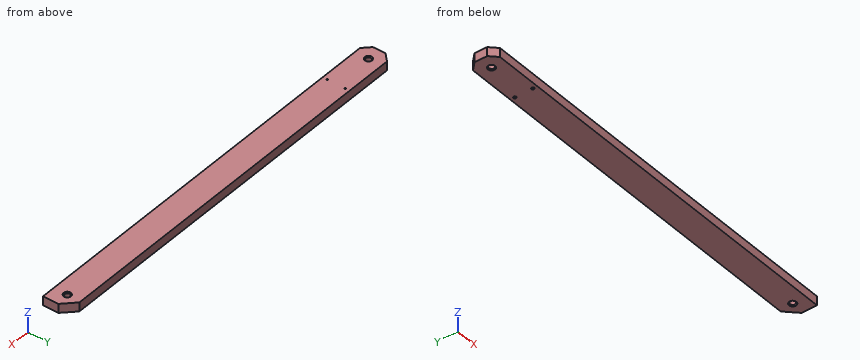
Autodesk Inventor part; units mm, degrees
ref_plane "YZ Plane" through (0, 0, 0) normal (1, 0, 0) x (0, 1, 0)
ref_plane "XZ Plane" through (0, 0, 0) normal (0, 1, 0) x (-1, 0, 0)
ref_plane "XY Plane" through (0, 0, 0) normal (0, 0, 1) x (1, 0, 0)
sketch "Sketch1" plane through (0, 0, 0) normal (0, 0, 1) x (1, 0, 0)
  line L0 (0, 0) -> (2250, 0)
  line L1 (2250, 0) -> (2250, 150)
  line L2 (2250, 150) -> (0, 150)
  line L3 (0, 150) -> (0, 0)
  dimension "d0" = 150
  dimension "d1" = 2250
extrude "Extrusion1" add sketch "Sketch1" along normal blind 50
sketch "Sketch2" plane through (0, 0, 50) normal (0, 0, 1) x (1, 0, 0)
  line L0 (0, 150) -> (0, 0)
  line L1 (2250, 0) -> (2250, 150)
  point P0 (75, 75)
  point P1 (2175, 75)
  point P2 (0, 75)
  dimension "d4" = 75
  dimension "d5" = 75
hole "Hole1" at (75, 75, 50) at (2175, 75, 50) direction (0, 0, -1) diameter 30 end through all
chamfer "Chamfer1" distance 5 angle 45 4 edges at (75, 90, 50) (2175, 90, 50) (75, 90, 0) (2175, 90, 0)
chamfer "Chamfer2" distance 65 angle 45 1 edges at (2250, 150, 25) measured on face at (2250, 50, 16.6667)
chamfer "Chamfer3" distance 40 angle 45 2 edges at (0, 150, 25) (0, 0, 25)
sketch "Sketch3" plane through (0, 0, 0) normal (0, 0, -1) x (-1, 0, 0)
  line L0 (-40, 0) -> (-2250, 0)
  line L1 (-2185, 150) -> (-40, 150)
  line L2 (0, 110) -> (0, 40)
  point P0 (0, 0)
  point P1 (-300, 25)
  point P2 (-300, 125)
  dimension "d22" = 25
  dimension "d23" = 25
  dimension "d24" = 300
hole "Hole2" at (300, 25, 0) at (300, 125, 0) direction (0, 0, 1) diameter 8.433 end through all countersink diameter 16.129 countersink angle 82
properties part number "Top_Rear Plank_LHS" material "Wood (Birch)"
The model under review builds one solid part; all positions refer to its coordinate system, in mm. Give positions to 0.01 mm unless a question says otherwise; leave off trailing zeros. Order: outer loops, then holes, each group sorted by start corner. A loop starts at its lowest first (then second) coordinate and runs counter-clockwise, first axis right, second up. Notation, with made-up numbers: M 29.5,48 L 46.5,48 A9 cw 46.5,60 Z; hole C 0,27 d2. An arc over 180 degrees is marked long. One line per question, with ' | ' between items. Start each with the question number.
1) Clearance check with flat-ended pins moving along their axes: P1, Ø1, axis at y = 111, z = 36, coming from the +X side; P2, Ø5, axis at x = 300, y = 125, coming from the +Z side; P3, Ø1.5, axis at y = 133.5, z = 17.5, coming from the +X side; P4, Ø2, axis at y = 115, z = 12, coming from the +X side. State where each tip first meets the part, or that it passes through.
2) Wall thickness on L1, parallel to Y at x = 300, z = 25.5; L2, parallel to X at y = 75, z = 28; L3, parallel to X at y = 80.5, z = 46.5: over which ranges is each line inside the solid? List them lowest first. Write a range as from..to.
3) Consider section A-A, the plane z = 26.5. Give the boundary of the cut face in (x, y).
Found:
1) P1: stops at x = 2224.5 | P2: passes through | P3: stops at x = 2202.25 | P4: stops at x = 2221
2) L1: y = 0..20.78, 29.22..120.78, 129.22..150 | L2: x = 0..60, 90..2160, 2190..2250 | L3: x = 0..59.44, 90.56..2159.44, 2190.56..2250
3) outline: M 0,40 L 40,0 L 2250,0 L 2250,85 L 2185,150 L 40,150 L 0,110 Z; hole C 75,75 d30; hole C 300,25 d8.43; hole C 300,125 d8.43; hole C 2175,75 d30
